Study the drawing (mm; zero at the part's minimum x, y, z) and answer. A direction names the side the tool comes from. Coordinates: 2 decimals unless noted, no trailing zeros. Write each loop counter-clockwise with the first axis right and the second up, starting at its lowest first coordinate (ties: lowest second). Pieces come first, ordered by that corner, then holes. Notation, with made-up numbers: (83, 73.25) -> (100, 73.25) arc R33 ccw to (100, 106.25) -> close; hole circle Ø6 at (-21.75, -21.5). An arc over 180 degrees is marked (long way). Write item = value, one per line. Start each with the question number.
1) Section A-A (y = 5) is taken. Determine the outline of the cut face in (x, z), plus the area to 3 significant figures.
2) Find the intervals of material crossed by line 1 along X through (y, z) = (4.75, 27.5); line 2 along Z through (x, y) = (6, 8); line 3 along X through (y, z) = (1, 21.5), in increasing order. Write a range as from..to.
3) A tool of negligible diameter and unlimited length cuts with its end or side. For the marked faces 1 and 2, from which of +Z, -Z, +X, -X, +Y, -Y can it reach the whole face along a straight path? Write none if from no direction.
4) Flat-ended cylindrical pins translate along their axes: pin 1 Ø5 at (x, z) = (3.5, 18) entering from +Y; pin 2 Ø2 at (x, z) = (2.5, 20) entering from -Y; pin 3 Ø3 at (x, z) = (5.5, 4.5) entering from -Y; pin 4 Ø1.3 at (x, z) = (5, 5.5) entering from +Y. Find the tip coordinate at first contact, or state that the pin passes through.
5) Section C-C (z = 23.75) is taken. Determine the outline of the cut face in (x, y) (1 decimal).
6) Section D-D (y = 8) is taken. Determine the outline of the cut face in (x, z), plus the area to 3 significant figures.
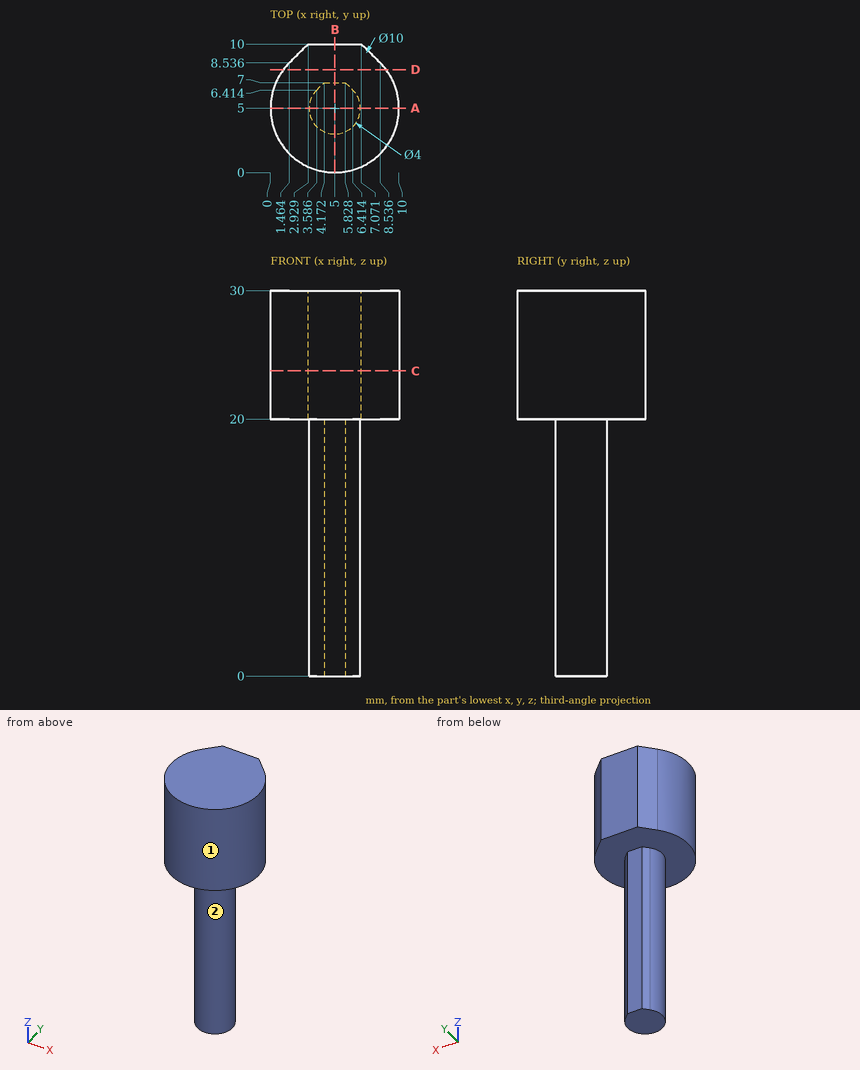
Answer key:
q1.outline = (0, 20) -> (3, 20) -> (3, 0) -> (7, 0) -> (7, 20) -> (10, 20) -> (10, 30) -> (0, 30) -> close
q1.area = 180 mm^2
q2.line_1 = 0.01..9.99
q2.line_2 = 20..30
q2.line_3 = 2..8
q3.face_1 = +Z, -Z
q3.face_2 = -Z
q4.pin_1 = 10
q4.pin_2 = 0.23
q4.pin_3 = 3
q4.pin_4 = 7
q5.outline = (1.5, 8.5) arc R5 ccw (long way) to (8.5, 8.5) -> (7.1, 10) -> (2.9, 10) -> close
q6.outline = (1, 20) -> (9, 20) -> (9, 30) -> (1, 30) -> close
q6.area = 80.0 mm^2
